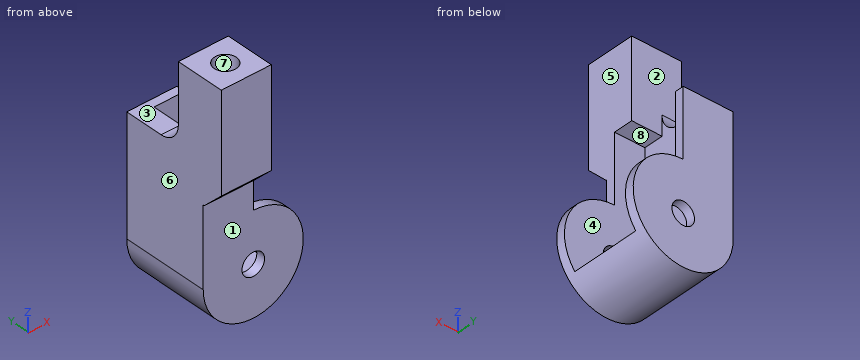
Autodesk Inventor part; units mm, degrees
ref_plane "YZ Plane" through (0, 0, 0) normal (1, 0, 0) x (0, 1, 0)
ref_plane "XZ Plane" through (0, 0, 0) normal (0, 1, 0) x (-1, 0, 0)
ref_plane "XY Plane" through (0, 0, 0) normal (0, 0, 1) x (1, 0, 0)
sketch "スケッチ1" plane through (0, 0, 0) normal (0, 1, 0) x (-1, 0, 0)
  circle A0 centre (0, 0) radius 1.15
  circle A1 centre (0, 0) radius 3.1
  circle A2 centre (0, 0) radius 5.1
  line L0 (3.1, 0) -> (5.1, 0)
  line L1 (5.1, 0) -> (5.1, 10)
  line L2 (5.1, 10) -> (3.1, 10)
  line L3 (3.1, 10) -> (3.1, 0)
  line L4 (0, 3.1) -> (3.1, 3.1)
  line L5 (5.1, 0) -> (1.8843, -2.4616)
  line L6 (5.1, 10) -> (0, 10)
  line L7 (0, 10) -> (0, 20)
  line L8 (0, 20) -> (5.1, 20)
  line L9 (5.1, 20) -> (5.1, 10)
  line L10 (0, 10) -> (0, 0)
  line L11 (0, -3.1) -> (-4.0497, -3.1)
  line L12 (3.1, 10) -> (5.1, 10)
  line L13 (5.1, 10) -> (5.1, 12)
  line L14 (5.1, 12) -> (3.1, 12)
  line L15 (3.1, 12) -> (3.1, 10)
  line L16 (3.1, 12) -> (0, 12)
  line L17 (0, 12) -> (0, 10)
  line L18 (0, 10) -> (3.1, 10)
  line L19 (3.1, 10) -> (3.1, 12)
  line L20 (0, 12) -> (5.1, 12)
  line L21 (5.1, 12) -> (5.1, 8)
  line L22 (5.1, 8) -> (0, 8)
  line L23 (0, 8) -> (0, 12)
  point P0 (0, 5.1)
  dimension "d2" = 10.2
  dimension "d0" = 2.3
  dimension "d1" = 6.2
  dimension "d3" = 10
  dimension "d4" = 10
  dimension "d7" = 2
  dimension "d8" = 2
  dimension "d22" = 4
extrude "押し出し1" add sketch "スケッチ1" along normal blind 7.1 contours L0 L5 A1 | L3 A2 L0 | A1 L5 A2 L11 | A2 L3 L22 L1 | L22 L3 L2 L1 | L2 L15 L14 L9
extrude "押し出し2" add sketch "スケッチ1" against normal blind 0.9
sketch "スケッチ2" plane through (0, 7.1, 0) normal (0, 1, 0) x (1, 0, 0)
  circle A0 centre (0, 0) radius 1.15
  circle A1 centre (0, 0) radius 3.1
  circle A2 centre (0, 0) radius 5.1
  line L0 (0, -12) -> (-5.1, -12)
  line L1 (0, 0) -> (-5.1, 0)
  line L2 (-5.1, 0) -> (-5.1, -12)
  line L3 (-5.1, -12) -> (0, -12)
  line L4 (0, -12) -> (0, 0)
  point P0 (0, -5.1)
  dimension "d11" = 2.3
  dimension "d12" = 6.2
  dimension "d13" = 10.2
  dimension "d14" = 5.1
  dimension "d15" = 12
extrude "押し出し3" add sketch "スケッチ2" along normal blind 0.9 contours A0 L1 A1 L4 | A0 L4 A1 L1 | L1 A2 L4 A1 | A1 L4 A2 L1 | A2 L4 L0 L2
extrude "押し出し4" add sketch "スケッチ1" along normal blind 2 contours L7 L8 L9 L14 L16
extrude "押し出し5" add sketch "スケッチ1" against normal blind 3 contours L10 L6 L3 L22 | L22 L3 L2 L1 | L7 L16 L15 L6 | L2 L15 L14 L9 | L7 L8 L9 L14 L16
chamfer "面取り1" distance 2 angle 45 1 edges at (-2.55, -3, 8)
sketch "スケッチ3" plane through (-5.1, 2, 20) normal (0, 0, 1) x (1, 0, 0)
  line L0 (0, -5) -> (0, 0)
  line L1 (0, 0) -> (2.6, 0)
  line L2 (2.6, 0) -> (2.6, -2.5)
  line L3 (2.6, -2.5) -> (0, -2.5)
  line L4 (0, -2.5) -> (0, 0)
  circle A0 centre (2.6, -2.5) radius 1.125
  point P0 (5.1, -2)
  dimension "d26" = 2.6
  dimension "d27" = 2.5
  dimension "d28" = 2.25
hole "穴1" at (-2.5, -0.5, 20) direction (0, 0, -1) diameter 2.25 depth 7
fillet "フィレット1" radius 2 1 edges at (-4.1, 2, 12)
properties part number "srod2.5_2.25"
Verification items for the finished model (mm, model axes). Face numbers are marked on the shaded views. A direction names the side the tool comes from. Coordinates: 2 decimals unless noted, no trailing zeros. Write each loop counter-clockwise with the first axis right and the second up, starting at its lowest first coordinate (ties: lowest second). Pieces come first, ordered by that corner, then holes. Notation, with made-up numbers: M -2.75,10 L 30.25,10 A28 cw 30.25,32 Z; hole C -37,39 d7. An arc over 180 degrees is marked long. One line per item, written item: value.
Item 1: Section check A-A, the plane y = -0.5. Record the boundary of the cut face in (x, z) (3 decimals), plus the area to 3 significant figures.
Check sheet entries:
outline: M -5.1,0 A5.1 ccw long 0,5.1 L 0,20 L -1.375,20 L -1.375,13 L -3.625,13 L -3.625,20 L -5.1,20 Z; hole C 0,0 d2.3
area: 143 mm^2
Item 2: Section check C-C, the plane y = 1.5. Record the boundary of the cut face in (x, z), plus the area to 3 significant figures.
Check sheet entries:
outline: M -5.1,0 A5.1 ccw 4.05,-3.1 L 0,-3.1 A3.1 cw -3.1,0 L -3.1,12 L 0,12 L 0,20 L -5.1,20 Z
area: 83.3 mm^2
Item 3: Section check D-D, the plane x = -2.5. Record the boundary of the cut face in (y, z) (3 decimals).
Check sheet entries:
outline: M -3,10 L -1,8 L -0.9,8 L -0.9,-4.445 L 8,-4.445 L 8,12 L 7.1,12 L 7.1,-1.833 L 0,-1.833 L 0,12 L 2,12 L 2,20 L 0.625,20 L 0.625,13 L -1.625,13 L -1.625,20 L -3,20 Z
Item 4: Gauge pin test, flat ends, axial feed: pin 1 Ø4 at (y, z) = (-1.5, 9.5) entering from +X; pin 2 Ø3 at (x, z) = (0, 0) entering from -Y; pin 3 Ø4 at (x, z) = (-3.5, 17) entering from +Y; pin 4 Ø4 at (x, y) = (0.5, 1) entering from -Z. Record the tip position at first contact, or that the pin passes through.
Check sheet entries:
pin 1: stops at x = 0
pin 2: stops at y = -0.9
pin 3: stops at y = 2
pin 4: stops at z = -5.1
Item 5: Access from +Z, -Z, +X, -X, +Y, -Y to the whole of each face (thin tool, end or side, straight path). Record for the marked faces 1, 2, 3 and 4.
Check sheet entries:
face 1: -Z, +X, -X, -Y
face 2: +Z, +X, +Y
face 3: +Z, +X, -X, +Y
face 4: +X
Item 6: Mould release check, pull along X, two halves, no side actions. Record for the marked faces 5, 6, 7 and 8: pulls with the +X half, pulls with the -X half, needs draft (parallel to the pull), parting line crosses it, or undercut.
Check sheet entries:
face 5: pulls with the +X half
face 6: pulls with the -X half
face 7: undercut
face 8: needs draft
Item 7: Scan lines: line 1 along X through (y, z) = (-0.35, 0); line 2 along Y through (x, z) = (-1.75, 2); line 3 along Y through (x, z) = (-2.5, 16.5) (3 decimals). Record each from-to range of solid material in increasing order.
Check sheet entries:
line 1: x = -5.1 to -1.15, 1.15 to 5.1
line 2: y = -0.9 to 0, 7.1 to 8
line 3: y = -3 to -1.625, 0.625 to 2
Item 8: Section check B-B, the plane x = 1.5. Record the boundary of the cut face in (y, z), plus the area to 3 significant figures.
Check sheet entries:
outline: M -0.9,-4.87 L 8,-4.87 L 8,4.87 L 7.1,4.87 L 7.1,-3.1 L 0,-3.1 L 0,4.87 L -0.9,4.87 Z
area: 30.1 mm^2
